The listing builds one solid part. Answer for the finished solid, in the listing's coordinates (mm). Face numbers are marked on the shaded views. Coordinates: 2 decimals unless noted, no trailing zeros. Loops run counter-clockwise (first coordinate to the right, second up) from the corner with the lowest first, then second, coordinate; pieces in that order, holes last. Notation, with made-up numbers: (26, -24.5) - (56, -24.5) arc R28 cw to (56, -5.5) - close; hole circle Ø10 at (43.25, 6). An arc over 180 degrees is marked (long way). Return JSON: item names as keys, results as strings. Group by question number.
1. Section A-A (z = -3.5) is taken. Write down the section's boundary in (x, y), and give its area (3 significant figures).
2. Section D-D (z = -23.5) is taken. Write down the section's boundary in (x, y).
3. Section B-B (y = 1.95) is taken. State how many separate pieces and enclosed holes the cut face has, and give its area (3 significant figures).
4. Section C-C (x = 12.7) is taken. Write down the section's boundary in (y, z).
5. This flat-tipped pin is pushed along its axis until it touches: P1, Ø1, axis at x = 13, y = 2, coming from the +Z side. Where does it stop, or does it pass through?
6. The mould has two halves that part along X. Classify the marked faces 1, 2, 3 and 4: pulls with the +X half, pulls with the -X half, needs draft (parallel to the pull), parting line crosses it, or undercut.
7. Find the intervals of material crossed by line 1 along Z through (x, y) = (6.5, 1.65); line 2 along X through (y, z) = (2.55, -12.7); line 3 along Z through (x, y) = (20.25, 2.6), in increasing order.
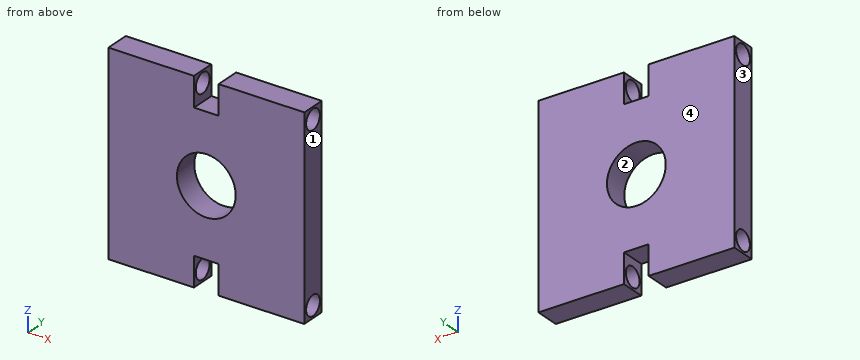
```python
from build123d import *

# Parameters (mm, degrees)
SKETCH1_R           = 3.81
BOSS_EXTRUDE1_DEPTH = 3.2004
SKETCH3_R           = 1.27
CUT_EXTRUDE2_DEPTH  = 37.063313217


with BuildPart() as part:
    # Sketch1 → Boss-Extrude1 (new body)
    with BuildSketch(Plane(origin=(0, 0, 0), x_dir=(1, 0, 0), z_dir=(0, 1, 0))):
        Polygon((0, 25.4), (11.0998, 25.4), (11.0998, 21.59), (14.3002, 21.59), (14.3002, 25.4), (25.4, 25.4), (25.4, 0), (14.3002, 0), (14.3002, 3.81), (11.0998, 3.81), (11.0998, 0), (0, 0), align=None)
        with Locations(Location((12.7, 12.7, 0), (0, 0, 270))):
            Circle(SKETCH1_R, mode=Mode.SUBTRACT)
    extrude(amount=BOSS_EXTRUDE1_DEPTH)

    # Sketch3 → Cut-Extrude2 (cut, through all)
    with BuildSketch(Plane(origin=(25.4, 0, 0), x_dir=(0, 0, -1), z_dir=(1, 0, 0))):
        with Locations((23.860164918, 1.6002)):
            Circle(SKETCH3_R)
        with Locations((1.539835082, 1.6002)):
            Circle(SKETCH3_R)
    extrude(amount=-CUT_EXTRUDE2_DEPTH, mode=Mode.SUBTRACT)


solid = part.part
```
The answers:
{
 "1": {"outline": "(0, 0) - (11.1, 0) - (11.1, 3.2) - (0, 3.2) - close; (14.3, 0) - (25.4, 0) - (25.4, 3.2) - (14.3, 3.2) - close", "area": "71.0 mm2"},
 "2": {"outline": "(0, 0) - (11.1, 0) - (11.1, 0.38) - (0, 0.38) - close; (0, 2.82) - (11.1, 2.82) - (11.1, 3.2) - (0, 3.2) - close; (14.3, 0) - (25.4, 0) - (25.4, 0.38) - (14.3, 0.38) - close; (14.3, 2.82) - (25.4, 2.82) - (25.4, 3.2) - (14.3, 3.2) - close"},
 "3": {"separate pieces": "5", "enclosed holes": "1", "area": "467 mm2"},
 "4": {"outline": "(0, -21.59) - (3.2, -21.59) - (3.2, -16.51) - (0, -16.51) - close; (0, -8.89) - (3.2, -8.89) - (3.2, -3.81) - (0, -3.81) - close"},
 "5": {"P1": "stops at z = -3.81"},
 "6": {"face 1": "pulls with the +X half", "face 2": "undercut", "face 3": "pulls with the -X half", "face 4": "needs draft"},
 "7": {"line 1": "z = -25.4 to -25.13, -22.59 to -2.81, -0.27 to 0", "line 2": "x = 0 to 8.89, 16.51 to 25.4", "line 3": "z = -25.4 to -24.64, -23.08 to -2.32, -0.76 to 0"}
}
